Source: CAD feature listing. Evaluate the final solid. Frame: model axes, mm. Face numbers are marked on the shaded views. A direction names the side the tool comes from. Round coordinates to 2 decimals unless told otherwise and drop trailing zeros. Loops run counter-clockwise (first coordinate to the right, second up) from the corner with the lowest first, then second, coordinate; pieces in that order, holes last.
(1) Section A-A, the plane x = 0. Return the cut outline in (y, z).
(2) Material intervals for probe 1 along Z at (x, y) = (0, -2.05); probe 2 along Y at (x, z) = (0, -2.1); probe 3 along Y at (x, z) = (5.75, -25.5), sorted ascending.
(3) Section B-B, the plane z = -15. Return the cut outline in (x, y), plus the area to 3 significant figures.
(4) Set-up query: the marked faces 1 and 2. Return all of +Z, -Z, +X, -X, +Y, -Y with unobstructed straight access to the full face (end or side cutting, diameter ignored); none if empty.
(5) First-contact query: pin 1 Ø10 at (x, z) = (-3.5, -10.5) entering from -Y; pin 2 Ø6 at (x, z) = (-7, -16) entering from +Y; pin 3 Ø10 at (x, y) = (6, -12.5) entering from -Z. Flat tips, straight axial feed; report the tip coordinate or a pass-through.
(6) Section D-D, the plane x = 3. Return the cut outline in (y, z), plus the area to 3 significant figures.
(7) Mould query, pull axis Y, two halves, no side actions, for the marked faces 3, 4 and 5. Classes: pulls with the +Y half, pulls with the -Y half, needs draft (parallel to the pull), parting line crosses it, or undercut.
```python
from build123d import *

# Parameters (mm, degrees)
F1_DEPTH = 10
F2_R     = 3.5
F3_DEPTH = 30.001
F4_R     = 3.5
F5_DEPTH = 30.001


with BuildPart() as f1:
    # F0 (on Right) → F1 (new body, symmetric)
    with BuildSketch(Plane.YZ):
        Polygon((0, 0), (-30, 0), (-30, -3), (-3, -3), (-3, -30), (0, -30), align=None)
    extrude(amount=F1_DEPTH, both=True)

    # F2 (on face) → F3 (cut, through all)
    with BuildSketch(Plane(origin=(0, 0, 0), x_dir=(-1, 0, 0), z_dir=(0, 1, 0))):
        with Locations((0, -15)):
            Circle(F2_R)
    extrude(amount=-F3_DEPTH, mode=Mode.SUBTRACT)

    # F4 (on face) → F5 (cut, through all)
    with BuildSketch(Plane.XY):
        with Locations((0, -20)):
            Circle(F4_R)
    extrude(amount=-F5_DEPTH, mode=Mode.SUBTRACT)


solid = f1.part
```
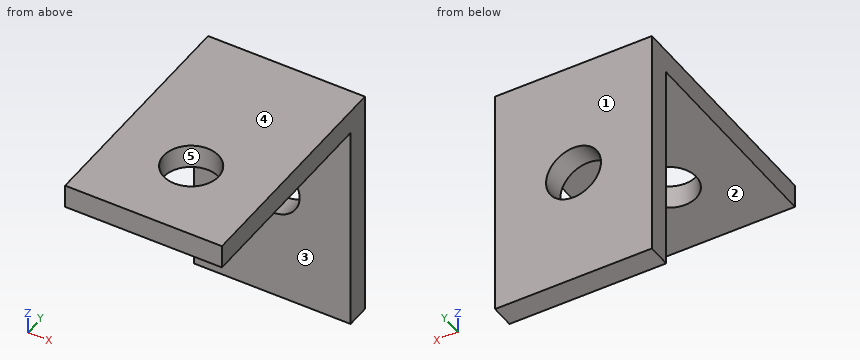
Output values:
1. outline: (-30, -3) - (-23.5, -3) - (-23.5, 0) - (-30, 0) - close; (-16.5, -3) - (-3, -3) - (-3, -11.5) - (0, -11.5) - (0, 0) - (-16.5, 0) - close; (-3, -30) - (0, -30) - (0, -18.5) - (-3, -18.5) - close
2. probe 1: z = -30 to -18.5, -11.5 to 0
2. probe 2: y = -30 to -23.5, -16.5 to 0
2. probe 3: y = -3 to 0
3. outline: (-10, -3) - (-3.5, -3) - (-3.5, 0) - (-10, 0) - close; (3.5, -3) - (10, -3) - (10, 0) - (3.5, 0) - close
3. area: 39.0 mm2
4. face 1: +Z, -Z, +X, -X, +Y
4. face 2: -Z, +X, -X, -Y
5. pin 1: stops at y = -3
5. pin 2: stops at y = 0
5. pin 3: stops at z = -3
6. outline: (-30, -3) - (-21.8, -3) - (-21.8, 0) - (-30, 0) - close; (-18.2, -3) - (-3, -3) - (-3, -13.2) - (0, -13.2) - (0, 0) - (-18.2, 0) - close; (-3, -30) - (0, -30) - (0, -16.8) - (-3, -16.8) - close
6. area: 149 mm2
7. face 3: pulls with the -Y half
7. face 4: needs draft
7. face 5: undercut
